Check sheet for the drawn part. Datum: minimum x, y, z corner. Units: mm. A direction names the side the tool comes from. Round coordinates to 2 decimals unless told otherwise and drop trailing zeros. Loops run counter-clockwise (first coordinate to the right, second up) from the corner with the lowest first, then second, coordinate; pieces in that order, holes last.
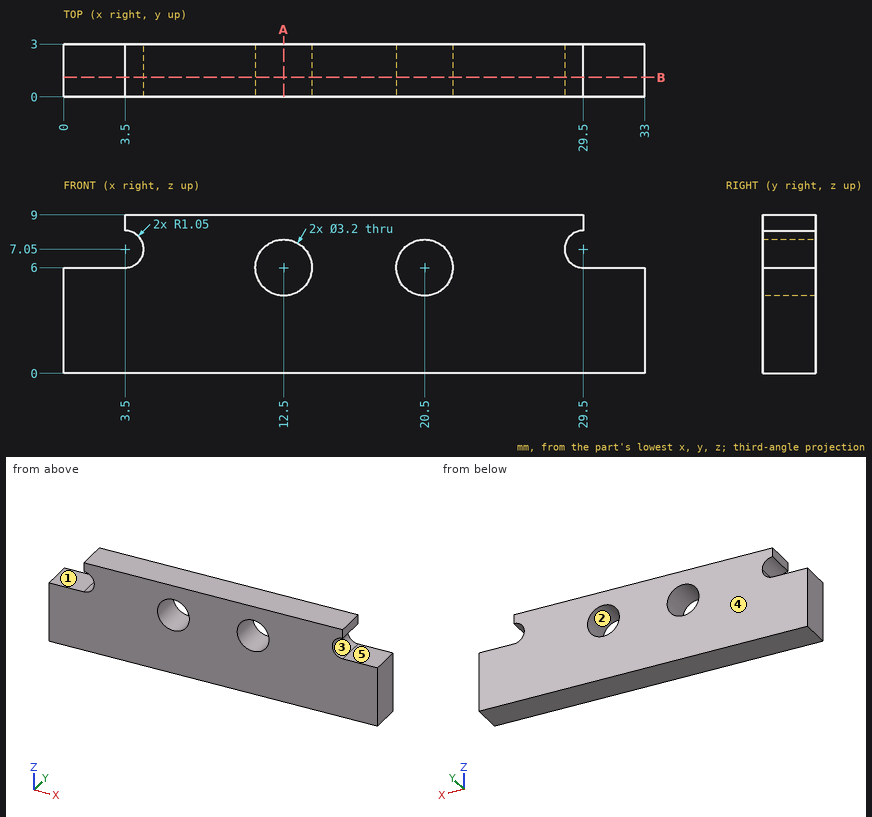
1. Section check A-A (x = 12.5). Enter the section's corners in (y, z).
2. Release check for a two-part mould opening along Z. For the marked faces 3, 4 and 5 record: released by +Z, released by -Z, zero draft, split by the parting line, or undercut.
3. Scan lines: L1, parallel to Z at x = 31, y = 2; L2, parallel to X at y = 2.45, z = 4.75; L3, parallel to Z at x = 13, y = 1.5. Record each from-to range of solid material in increasing order.
4. Section check B-B (y = 1.1). Enter the section's corners in (x, z).
5. Tool access check on the marked faces 1 and 2. Record the directions out of +Z, -Z, +X, -X, +Y, -Y that give a thin tool (end or side, any length) a straight path to the whole face; none if there is none.
6. Gauge pin test, flat ends, axial feed: P1, Ø4, axis at x = 12.5, z = 6, coming from the +Y side; P2, Ø1.5, axis at x = 32, y = 2, coming from the +Z side. Record the tip position at first contact, or that the pin passes through.
Taken from the geometry:
1. outline: (0, 0) - (3, 0) - (3, 4.4) - (0, 4.4) - close; (0, 7.6) - (3, 7.6) - (3, 9) - (0, 9) - close
2. face 3: undercut
2. face 4: zero draft
2. face 5: released by +Z
3. L1: z = 0 to 6
3. L2: x = 0 to 11.5, 13.5 to 19.5, 21.5 to 33
3. L3: z = 0 to 4.48, 7.52 to 9
4. outline: (0, 0) - (33, 0) - (33, 6) - (29.5, 6) arc R1.05 cw to (29.5, 8.1) - (29.5, 9) - (3.5, 9) - (3.5, 8.1) arc R1.05 cw to (3.5, 6) - (0, 6) - close; hole circle Ø3.2 at (12.5, 6); hole circle Ø3.2 at (20.5, 6)
5. face 1: +Z, -X, +Y, -Y
5. face 2: +Y, -Y
6. P1: stops at y = 3
6. P2: stops at z = 6
